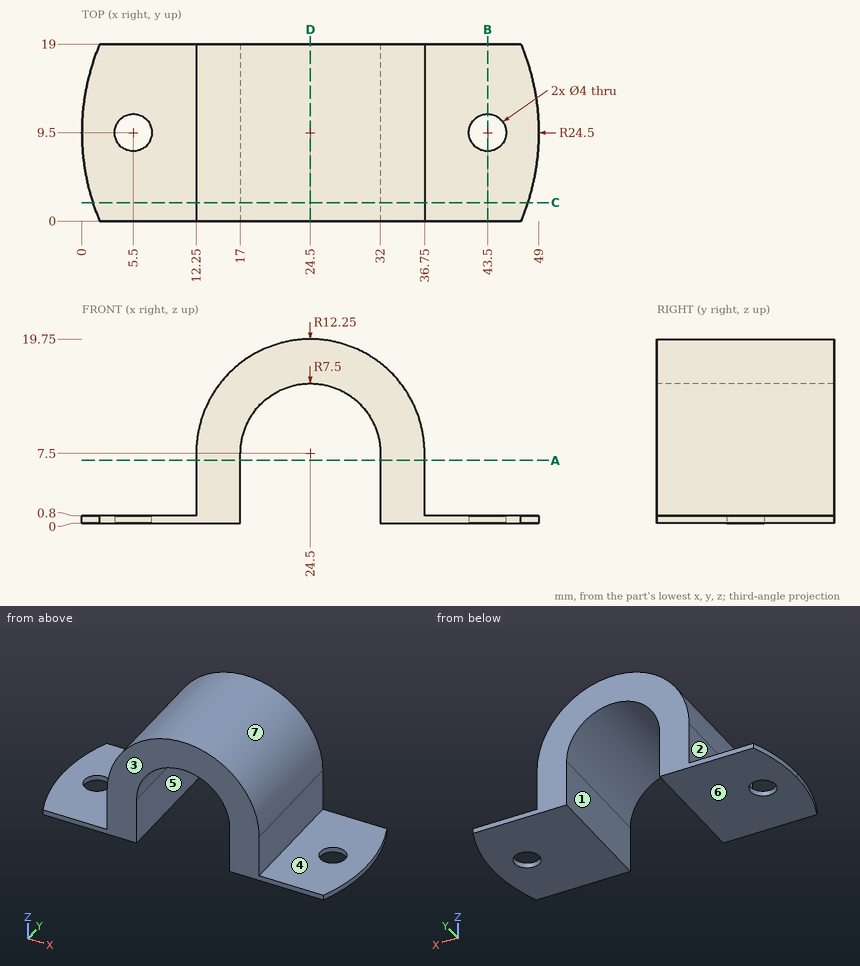
Geometry: see drawing. Coordinates: mm, zero at the bounding-box minimum. A direction names the side the tool comes from. Round coordinates to 2 decimals unless told otherwise and drop trailing zeros. Loops run counter-clockwise (first coordinate to the right, second up) from the corner with the lowest first, then second, coordinate; pieces in that order, holes last. Notation, with made-up numbers: M 5,31.5 L 21,31.5 A15 ccw 21,57.5 Z; hole C 61,88.5 d6. An arc over 180 degrees is marked long. Use a Markdown table: item, result. Add a question column.
1. Section query A-A on z = 6.75. Return the cut outline in (x, y).
2. Section query B-B on x = 43.5. Return the cut outline in (y, z), then the cut area to 3 significant figures.
3. Section query D-D on x = 24.5. Return the cut outline in (y, z).
4. Mould query, pull axis X, two halves, no side actions, for the marked faces 5, 6 and 7. Classes: pulls with the +X half, pulls with the -X half, needs draft (parallel to the pull), parting line crosses it, or undercut.
5. Line query: line 1 (X direction, y = 6, z = 2.5); line 2 (Y direction, x = 43.5, z = 0.3); line 3 (Z direction, x = 46.5, y = 2.5). Output: solid intervals per line, ascending.
6. Reachability of the marked faces 1, 2, 3 and 4 from +Z, -Z, +X, -X, +Y, -Y: full face, straight path, thin tool, end or side. Return the list, or none.
7. Section query C-C on y = 2. Return the cut outline in (x, z), then the cut area to 3 significant figures.
8. Contact query for flat-ended pins moving along their axis: P1, Ø6, axis at x = 12, y = 16, coming from the +Z side; P2, Ø10, axis at x = 42, y = 7, coming from the +Z side; P3, Ø3.5, axis at x = 43.5, y = 9.5, coming from the +Z side; P4, Ø8, axis at y = 7, z = 6.5, coming from the +X side. Output: stop coordinate, or through.
Reported:
| question | item | result |
|---|---|---|
| 1 | outline | M 12.25,0 L 17,0 L 17,19 L 12.25,19 Z; M 32,0 L 36.75,0 L 36.75,19 L 32,19 Z |
| 2 | outline | M 0,0 L 7.5,0 L 7.5,0.8 L 0,0.8 Z; M 11.5,0 L 19,0 L 19,0.8 L 11.5,0.8 Z |
| 2 | area | 12.0 mm² |
| 3 | outline | M 0,15 L 19,15 L 19,19.75 L 0,19.75 Z |
| 4 | face 5 | undercut |
| 4 | face 6 | needs draft |
| 4 | face 7 | parting line crosses it |
| 5 | line 1 | x = 12.25 to 17, 32 to 36.75 |
| 5 | line 2 | y = 0 to 7.5, 11.5 to 19 |
| 5 | line 3 | z = 0 to 0.8 |
| 6 | face 1 | -Z, +Y, -Y |
| 6 | face 2 | +Z, -X, +Y, -Y |
| 6 | face 3 | +Z, -Z, +X, -X, -Y |
| 6 | face 4 | +Z, +X, +Y, -Y |
| 7 | outline | M 1.18,0 L 17,0 L 17,7.5 A7.5 cw 32,7.5 L 32,0 L 47.82,0 L 47.82,0.8 L 36.75,0.8 L 36.75,7.5 A12.25 ccw 12.25,7.5 L 12.25,0.8 L 1.18,0.8 Z |
| 7 | area | 236 mm² |
| 8 | P1 | stops at z = 15.23 |
| 8 | P2 | stops at z = 0.8 |
| 8 | P3 | passes through |
| 8 | P4 | stops at x = 36.75 |
